Here's how the part is built. I have some questions about the finished solid (model axes, mm). A direction names the side the tool comes from. Give positions to 0.01 mm unless a question says otherwise; leave off trailing zeros. Write each loop counter-clockwise with the first axis right and the second up, starting at its lowest first coordinate (ties: lowest second). Pieces come first, ordered by that corner, then holes. Notation, with made-up numbers: (-11, 7) -> (39, 7) arc R20 cw to (39, 35) -> close; hole circle Ø2 at (1.5, 75). An arc over 180 degrees is marked (long way). Use one line per item in the form item = value.
Autodesk Inventor part; units mm, degrees
ref_plane "hhpsjc_l_XY" through (0, 0, 0) normal (0, 1, 0) x (1, 0, 0)
ref_plane "hhpsjc_l_YZ" through (0, 0, 0) normal (1, 0, 0) x (0, 0, -1)
ref_plane "hhpsjc_l_ZX" through (0, 0, 0) normal (0, 0, -1) x (0, 1, 0)
sketch "Sketch_1" plane through (0, 0, 0) normal (0, 0, 1) x (1, 0, 0)
  line L0 (0, -16) -> (0, 16)
  line L1 (0, 16) -> (5, 16)
  line L2 (5, 16) -> (5, -16)
  line L3 (5, -16) -> (0, -16)
  line L4 (0, -16) -> (0, 16)
revolve "Revolution1" add sketch "Sketch_1" angle 360 about axis through (0, -16, 0) along (0, -1, 0)
sketch "Sketch_2" plane through (0, 0, 0) normal (0, 1, 0) x (-1, 0, 0)
  arc A0 (18, -5) -> (16, 1) centre (8, -5) ccw
  line L0 (16, 1) -> (0, 1)
  line L1 (0, 1) -> (0, -5)
  line L2 (0, -5) -> (18, -5)
extrude "Extrusion1" add sketch "Sketch_2" along normal mid plane 32
sketch "Sketch_3" plane through (0, 0, 0) normal (0, 0, 1) x (1, 0, 0)
  line L0 (-36, -36) -> (36, -36)
  line L1 (36, -36) -> (36, 36)
  line L2 (36, 36) -> (-36, 36)
  line L3 (-36, 36) -> (-36, -36)
  line L4 (-18, 12) -> (-18, -12)
  arc A0 (-18, -12) -> (-14, -16) centre (-14, -12) ccw
  line L5 (-14, -16) -> (-5, -16)
  line L6 (-5, -16) -> (-5, -5.1333)
  line L7 (-5, -5.1333) -> (5, -5.1333)
  line L8 (5, -5.1333) -> (5, 5.1333)
  line L9 (5, 5.1333) -> (-5, 5.1333)
  line L10 (-5, 5.1333) -> (-5, 16)
  line L11 (-5, 16) -> (-14, 16)
  arc A1 (-14, 16) -> (-18, 12) centre (-14, 12) ccw
extrude "Extrusion2" cut sketch "Sketch_3" along normal mid plane 10
sketch "Sketch_4" plane through (-18, 0, 0) normal (1, 0, 0) x (0, 0, -1)
  line L0 (-5, -32) -> (10, -32)
  line L1 (10, -32) -> (10, 32)
  line L2 (10, 32) -> (-5, 32)
  line L3 (-5, 32) -> (-5, -32)
  line L4 (-1, 14) -> (-1, -14)
  arc A0 (-1, -14) -> (5, -16) centre (5, -6) ccw
  line L5 (5, -16) -> (5, 16)
  arc A1 (5, 16) -> (-1, 14) centre (5, 6) ccw
extrude "Extrusion3" cut sketch "Sketch_4" along normal blind 13
sketch "Sketch_6" plane through (0, 0, -5) normal (0, 0, 1) x (1, 0, 0)
  circle A0 centre (-10.5, 12) radius 2.75
extrude "Extrusion4" add sketch "Sketch_6" against normal blind 4
sketch "Sketch_5" plane through (0, 0, -5) normal (0, 0, 1) x (1, 0, 0)
  circle A0 centre (-10.5, -12) radius 2.75
extrude "Extrusion5" add sketch "Sketch_5" against normal blind 4
sketch "Sketch_7" plane through (-10.5, 0, 0) normal (1, 0, 0) x (0, 0, -1)
  line L0 (5, 0) -> (-1, 0)
  line L1 (-1, 0) -> (-1, 5.5)
  line L2 (-1, 5.5) -> (1.75, 2.75)
  line L3 (1.75, 2.75) -> (5, 2.75)
  line L4 (5, 2.75) -> (5, 0)
  line L5 (5, 0) -> (-1, 0)
revolve "Revolution2" cut sketch "Sketch_7" angle 360 about axis through (-10.5, 0, -5) along (0, 0, -1)
sketch "Sketch_8" plane through (0, 0, 0) normal (0, 0, 1) x (1, 0, 0)
  line L0 (0, -16) -> (0, 16)
  line L1 (0, 16) -> (2.5, 16)
  line L2 (2.5, 16) -> (2.5, -16)
  line L3 (2.5, -16) -> (0, -16)
  line L4 (0, -16) -> (0, 16)
revolve "Revolution3" cut sketch "Sketch_8" angle 360 about axis through (0, -16, 0) along (0, -1, 0)
ref_plane "hhpsjc_l_XY" through (0, 0, 0) normal (0, 1, 0) x (1, 0, 0)
ref_plane "hhpsjc_l_YZ" through (0, 0, 0) normal (1, 0, 0) x (0, 0, -1)
ref_plane "hhpsjc_l_ZX" through (0, 0, 0) normal (0, 0, -1) x (0, 1, 0)
ref_plane "hole1_to_bolt_XY" through (-10.5, 0, 1) normal (0, 0, 1) x (1, 0, 0)
ref_plane "hole1_to_bolt_YZ" through (-10.5, 0, 1) normal (1, 0, 0) x (0, 1, 0)
ref_plane "hole1_to_bolt_ZX" through (-10.5, 0, 1) normal (0, 1, 0) x (0, 0, 1)
ref_plane "nut1_to_bolt_XY" through (-10.5, 0, -7) normal (0, 0, 1) x (1, 0, 0)
ref_plane "nut1_to_bolt_YZ" through (-10.5, 0, -7) normal (1, 0, 0) x (0, 1, 0)
ref_plane "nut1_to_bolt_ZX" through (-10.5, 0, -7) normal (0, 1, 0) x (0, 0, 1)
properties part number "HHPSJC5-125_l"
Q1. If I drill on line 1 along Z through (x, y) = (0, -0.25); line 2 along Y through (x, z) = (-4.5, -3.25); line 3 along Z through (x, y) = (-9, -10), over which ranges is the centre line in solid material (lowest first)? Write a range as from..to.
Result set:
line_1 = -5..-2.5, 2.5..5
line_2 = -5.13..5.13
line_3 = -9..1
Q2. I want a section at C-C, the plane z = 1.75. Write out the boundary of the cut face in (x, y).
Result set:
outline = (-4.68, -5.13) -> (-1.79, -5.13) -> (-1.79, 5.13) -> (-4.68, 5.13) -> close; (1.79, -5.13) -> (4.68, -5.13) -> (4.68, 5.13) -> (1.79, 5.13) -> close
Q3. I want a section at B-B, the plane y = 1. Count the separate pieces of the cut face and the enclosed holes in it, and give its area (3 significant figures).
Result set:
separate_pieces = 2
enclosed_holes = 1
area = 99.8 mm2
Q4. If we mould it in two halves opening along Y, with no side actions, what happens to faces 4 (the face through (-11, 12, -9)), 5 (the face through (-11, -15.5, -1.88)), 6 (the face through (-8.641, -2.027, -3.398)), 7 (the face through (-7.88, -11.17, -6.97))? For each: +Y half, -Y half, draft (parallel to the pull), parting line (faces both ways), or undercut.
Result set:
face_4 = draft
face_5 = -Y half
face_6 = undercut
face_7 = undercut
Q5. I want a section at D-D, the plane y = -6. Write out the boundary of the cut face in (x, z), and give its area (3 significant figures).
Result set:
outline = (-18, -5) -> (-5, -5) -> (-5, 1) -> (-16, 1) arc R10 ccw to start
area = 74.2 mm2
Q6. I want a section at A-A, the plane z = -4. Write out the boundary of the cut face in (x, y), and give its area (3 significant figures).
Result set:
outline = (-17.95, -12.63) arc R4 ccw to (-14.63, -15.95) -> (-5, -15.95) -> (-5, -5.13) -> (3, -5.13) -> (3, 5.13) -> (-5, 5.13) -> (-5, 15.95) -> (-14.63, 15.95) arc R4 ccw to (-17.95, 12.63) -> close; hole circle Ø5.5 at (-10.5, 0)
area = 465 mm2
Q7. Which directions (+Z, -Z, +X, -X, +Y, -Y) give clear straight access to the entire face, cutting with the end or side of a thin tool? Please do faces 1 (the face through (-7.88, 12.83, -6.97)), 2 (the face through (-5, -11, -2)), 3 (the face through (-2, 5.133, -2)).
Result set:
face_1 = -Z
face_2 = +Z, -Z, +X, -Y
face_3 = +Z, -Z, +X, +Y
Q8. Will these pins go through, and if not, where does the flat tip stop? pin 1 Ø3 at (x, z) = (-4.5, -3.5) entering from -Y; pin 2 Ø2 at (x, z) = (-4.5, -7) entering from -Y; pin 3 Ø5.5 at (x, y) = (-10.5, -2) entering from +Z; pin 4 Ø8 at (x, z) = (-8, 0) entering from +Y.
Result set:
pin_1 = -16
pin_2 = through
pin_3 = 0.25
pin_4 = 15.95
